from build123d import *

# Parameters (mm, degrees)
F0_R     = 76.231661
F1_DEPTH = 25.4


with BuildPart() as f1:
    # F0 (on Top) → F1 (new body)
    with BuildSketch(Plane.XY):
        Circle(F0_R)
        Polygon((-54.700378, -42.292298), (-63.378183, -20.53418), (-45.366573, -5.557469), (-25.55698, -18.05947), (-31.325589, -40.762842), align=None, mode=Mode.SUBTRACT)
        Polygon((9.276015, -68.518065), (-13.90597, -65.154207), (-17.870377, -42.067339), (2.861469, -31.162729), (19.638862, -47.510177), align=None, mode=Mode.SUBTRACT)
        Polygon((63.976393, -26.225768), (49.472213, -44.620026), (27.496196, -36.50987), (28.41845, -13.10326), (50.964451, -6.747335), align=None, mode=Mode.SUBTRACT)
        Polygon((-63.976393, 26.225768), (-49.472213, 44.620026), (-27.496196, 36.50987), (-28.41845, 13.10326), (-50.964451, 6.747335), align=None, mode=Mode.SUBTRACT)
        Polygon((-2.861469, 31.162729), (-19.638862, 47.510177), (-9.276015, 68.518065), (13.90597, 65.154207), (17.870377, 42.067339), align=None, mode=Mode.SUBTRACT)
        Polygon((54.700378, 42.292298), (63.378183, 20.53418), (45.366573, 5.557469), (25.55698, 18.05947), (31.325589, 40.762842), align=None, mode=Mode.SUBTRACT)
    extrude(amount=F1_DEPTH)


solid = f1.part
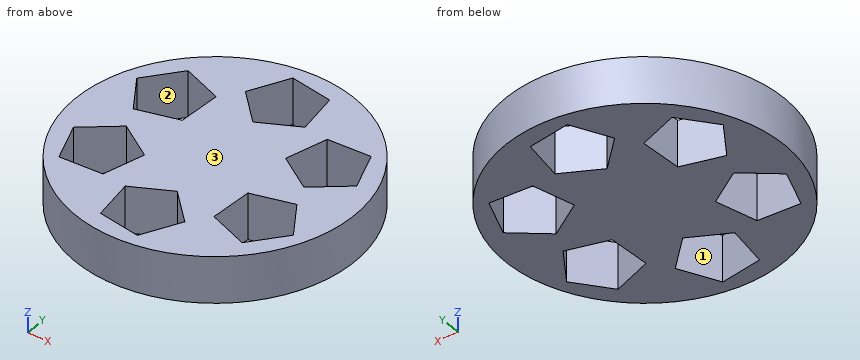
Model file for the job. Use its own axes, mm. Face numbers are marked on the shaded views. Coordinates: 2 decimals unless noted, no trailing zeros. Write each loop counter-clockwise with the first axis right and the second up, starting at its lowest first coordinate (ties: lowest second). Pieces come first, ordered by that corner, then holes. Notation, with made-up numbers: (-38.75, 62) -> (17.25, 62) arc R11 cw to (17.25, 68) -> close; hole circle Ø1 at (37, 74.5). An arc over 180 degrees is marked (long way). One line per item, written item: value. Start each with the question number.
1) Pull direction X, two halves, no side cores. Call the marked faces 1, 2 and 3: +X half, -X half, draft (parallel to the pull), parting line (faces both ways), or undercut.
2) Flat gauge pins, fed straight in: pin 1 Ø1.5 at (y, z) = (-17.5, 21.5) entering from +X; pin 2 Ø1 at (x, z) = (-56.5, 10.5) entering from +Y; pin 3 Ø3 at (x, z) = (-2.5, 20) entering from +Y. Where does each tip first touch, or does it go through?
3) Slice it at B-B on y = 57.5. Write the cut outline in (x, z), then the cut area to 3 significant figures.
4) Probe probe 1 along Y at (x, z) = (40, 17.25); probe 2 along Y at (x, z) = (-4, 3); probe 3 along X at (y, z) = (25, 14). List the from-to ranges inside material, lowest first.
5) Slice it at A-A on z = 1.75. Count the separate pieces of the cut face and the enclosed holes in it, then the cut area to 3 significant figures.
6) Slice it at D-D on y = -62.5. Write the cut outline in (x, z), then the cut area to 3 significant figures.
7) Slice it at C-C on x = 0. Write the cut outline in (y, z), then the cut area to 3 significant figures.
Answers follow:
1. face 1: undercut
1. face 2: undercut
1. face 3: draft
2. pin 1: x = 74.37
2. pin 2: y = 51.72
2. pin 3: y = 76.23
3. outline: (-50.05, 0) -> (-14.71, 0) -> (-14.71, 25.4) -> (-50.05, 25.4) -> close; (15.22, 0) -> (50.05, 0) -> (50.05, 25.4) -> (15.22, 25.4) -> close
3. area: 1,780 mm2
4. probe 1: -64.89 to -41.12, -9.84 to 8.94, 41.33 to 64.89
4. probe 2: -76.13 to -66.59, -34.77 to 32.27, 67.75 to 76.13
4. probe 3: -72.02 to -63.16, -27.95 to 27.32, 61.6 to 72.02
5. separate pieces: 1
5. enclosed holes: 6
5. area: 12,600 mm2
6. outline: (-43.65, 0) -> (-14.36, 0) -> (-14.36, 25.4) -> (-43.65, 25.4) -> close; (12.24, 0) -> (43.65, 0) -> (43.65, 25.4) -> (12.24, 25.4) -> close
6. area: 1,540 mm2
7. outline: (-76.23, 0) -> (-67.17, 0) -> (-67.17, 25.4) -> (-76.23, 25.4) -> close; (-32.67, 0) -> (32.67, 0) -> (32.67, 25.4) -> (-32.67, 25.4) -> close; (67.17, 0) -> (76.23, 0) -> (76.23, 25.4) -> (67.17, 25.4) -> close
7. area: 2,120 mm2
